Work out the finished part from the listing and answer in its coordinate system (mm). A direction names the side the tool comes from. Round coordinates to 2 decimals unless told otherwise and drop trailing zeros. Write each loop counter-clockwise with the first axis right and the second up, starting at its lowest first coordinate (ties: lowest second). Pieces come first, ordered by that corner, then holes. Notation, with made-up numbers: M 37,22.5 L 72,22.5 A21 ccw 72,56.5 Z; hole C -39.75,-38.5 d5. An arc over 180 degrees is marked long. One line per item, written item: value. Start each with the question number.
Q1. Find section C-C (y = -46). Write down the section's boundary in (x, z), and give its area (4 significant figures).
Q2. Consider probe 1 along Z at (x, y) = (0, 9.25); probe 2 along Y at (x, z) = (0, 4.75); probe 3 along Z at (x, y) = (3.75, -22.5). Determine where each line is inside the solid, lowest interval first.
Q3. Find section D-D (z = 14). Write down the section's boundary in (x, y).
Q4. The mould has two halves that part along Z. Classify faces 1 (the flat face through (0, 9, 78)), 2 (the cylindrical face through (-0.92, 8.87, 58.85)), 3 (the cylindrical face through (-0.8, -39.8, 7.6)): released by +Z, released by -Z, zero draft, split by the parting line, or undercut.
Q5. Find section A-A (z = 63). Write down the section's boundary in (x, y), and give its area (3 significant figures).
Q6. A tool of negligible diameter and unlimited length cuts with its end or side. For faces 4 (the flat face through (0, 18, 40)), 5 (the flat face through (0, -31, 15)), from which of +Z, -Z, +X, -X, +Y, -Y can it reach the whole face along a straight path? Write none if from no direction.
Q7. Find section B-B (x = 0). Write down the section's boundary in (y, z).
Q8. Given pin 1 Ø2 at (x, z) = (-9.5, 56.5) entering from -Y; pin 2 Ø7.5 at (x, y) = (-4.5, -25.5) entering from +Z; pin 3 Ø6 at (x, y) = (1, -45.5) entering from -Z, each flat-ended and moving along its own axis, determine where each tip first touches the part or whether it passes through.
from build123d import *

# Parameters (mm, degrees)
F0_W     = 25
F0_H     = 15
F0_H_2   = 63
F0_R     = 4.25
F1_DEPTH = 18
F2_DEPTH = 62
F3_R     = 6.25
F4_DEPTH = 25.4


with BuildPart() as f1:
    # F0 (on Front) → F1 (new body)
    with BuildSketch(Plane.XZ):
        with Locations((0, 7.5)):
            Rectangle(F0_W, F0_H)
        with Locations((0, 46.5)):
            Rectangle(F0_W, F0_H_2)
        with Locations((0, 29.5)):
            Circle(F0_R, mode=Mode.SUBTRACT)
        with Locations((0, 63)):
            Circle(F0_R, mode=Mode.SUBTRACT)
    extrude(amount=-F1_DEPTH)

    # F0 (on Front) → F2 (join)
    with BuildSketch(Plane.XZ):
        with Locations((0, 7.5)):
            Rectangle(F0_W, F0_H)
    extrude(amount=F2_DEPTH)

    # F3 (on face) → F4 (cut)
    with BuildSketch(Plane.XY.offset(15)):
        with Locations((0, -46)):
            Circle(F3_R)
    extrude(amount=-F4_DEPTH, mode=Mode.SUBTRACT)


solid = f1.part
The answers:
1. outline: M -12.5,0 L -6.25,0 L -6.25,15 L -12.5,15 Z; M 6.25,0 L 12.5,0 L 12.5,15 L 6.25,15 Z
1. area: 187.5 mm2
2. probe 1: 0 to 25.25, 33.75 to 58.75, 67.25 to 78
2. probe 2: -62 to -52.25, -39.75 to 18
2. probe 3: 0 to 15
3. outline: M -12.5,-62 L 12.5,-62 L 12.5,18 L -12.5,18 Z; hole C 0,-46 d12.5
4. face 1: released by +Z
4. face 2: undercut
4. face 3: zero draft
5. outline: M -12.5,0 L -4.25,0 L -4.25,18 L -12.5,18 Z; M 4.25,0 L 12.5,0 L 12.5,18 L 4.25,18 Z
5. area: 297 mm2
6. face 4: +Z, -Z, +X, -X, +Y
6. face 5: +Z, +X, -X, -Y
7. outline: M -62,0 L -52.25,0 L -52.25,15 L -62,15 Z; M -39.75,0 L 18,0 L 18,25.25 L 0,25.25 L 0,15 L -39.75,15 Z; M 0,33.75 L 18,33.75 L 18,58.75 L 0,58.75 Z; M 0,67.25 L 18,67.25 L 18,78 L 0,78 Z
8. pin 1: y = 0
8. pin 2: z = 15
8. pin 3: through
